Design review of the part built by this model. Coordinates are the model's own, in mm. A direction names the side the tool comes from. Coordinates: 2 decimals unless noted, no trailing zeros. Write each loop counter-clockwise with the first axis right and the second up, starting at its lowest first coordinate (ties: lowest second). Pieces come first, ordered by that corner, then holes.
Q1. For faces 1 (the flat face through (-17.58, 7.52, -11.09)), 2 (the flat face through (-28.001, 7.521, -11.476)), 3 (the flat face through (-12.3, 7.5, -3.8)), list the 3-axis set-ups (+Z, -Z, +X, -X, +Y, -Y) from which the entire face can be reached by the end or side of a thin tool; tool diameter is ignored.
Q2. Take a section at A-A, the plane x = -43. Write out the cut boundary in (y, z), plus the area to 3 significant figures.
Q3. For pin 1 Ø1.5 at (x, y) = (-40, 8) entering from -Z; pin 2 Ø1.5 at (x, y) = (-46.5, 7.5) entering from +Z; pin 3 Ø3 at (x, z) = (-23.15, -1.62) entering from -Y, all flat-tipped, find the tip position at first contact; note any pin that passes through.
Q4. Take a section at B-B, the plane y = 7.05. State how many separate pieces and enclosed holes the cut face has, plus the area to 3 significant figures.
Q5. For L1, parallel to X at y = 7.3, z = -9.25; L2, parallel to X at y = 6.2, z = -1.25; L3, parallel to Z at x = -38.5, y = 6.4, list the stretches that pass through material, from the lowest coordinate up.
Q6. The part is to be moulded in two halves that separate along Z. For faces 4 (the flat face through (-19.018, 7.521, -11.83)), 5 (the cylindrical face through (-21.785, 7.479, 8.289)), 6 (the flat face through (-29, 6, -2)), say which applies: released by +Z, released by -Z, zero draft, split by the parting line, or undercut.
from build123d import *

# Parameters (mm, degrees)
BOSS_EXTRUDE1_DEPTH   = 15
BOSS_EXTRUDE2_DEPTH   = 15
CIRPATTERN2_COUNT     = 13
CIRPATTERN2_ANGLE     = 170
F_1_0MM_DOWEL_HOLE1_D = 10
ESCALA1_SCALE         = 0.2


with BuildPart() as part:
    # Sketch1 → Boss-Extrude1 (new body)
    with BuildSketch(Plane(origin=(0, 0, 0), x_dir=(1, 0, 0), z_dir=(0, 1, 0))):
        with BuildLine():
            Line((-150, 15), (-47.696960071, 15))
            ThreePointArc((-47.696960071, 15), (50, 0), (-47.696960071, -15))
            Line((-47.696960071, -15), (-150, -15))
            ThreePointArc((-150, -15), (-165, 0), (-150, 15))
        make_face()
    extrude(amount=BOSS_EXTRUDE1_DEPTH)

    # Sketch2 → Boss-Extrude2 (add)
    with BuildSketch(Plane(origin=(0, 15, 0), x_dir=(1, 0, 0), z_dir=(0, 1, 0))):
        Polygon((49.877349569, 3.5), (60, 2), (60, -2), (49.877349569, -3.5), (50, 0), align=None)
    boss_extrude2 = extrude(amount=-BOSS_EXTRUDE2_DEPTH)

    # CirPattern2: Boss-Extrude2 ×13 about axis
    cirpattern2_axis = Axis((0, 0, 0), (0, 1, 0))
    for i in range(1, CIRPATTERN2_COUNT):
        add(boss_extrude2.rotate(cirpattern2_axis, i * CIRPATTERN2_ANGLE / (CIRPATTERN2_COUNT - 1)))

    # Ø1.0mm Dowel Hole1 (through all)
    with Locations(Plane(origin=(0, 15, 0), x_dir=(1, 0, 0), z_dir=(0, 1, 0))):
        with Locations((-150, 0), (0, 0)):
            Hole(F_1_0MM_DOWEL_HOLE1_D / 2)


with BuildPart() as part_1:
    # Escala1: scaled about (-28.934441086, 7.5, -2.022629068)
    add(part.part.scale(ESCALA1_SCALE).moved(Location((-23.147552869, 6, -1.618103254))))


solid = part_1.part
Responses:
1. face 1: -Z, +Y, -Y
1. face 2: +Y, -Y
1. face 3: +X, +Y, -Y
2. outline: (6, -4.62) - (9, -4.62) - (9, 1.38) - (6, 1.38) - close
2. area: 18.0 mm2
3. pin 1: stops at z = -4.62
3. pin 2: stops at z = 1.38
3. pin 3: stops at y = 6
4. separate pieces: 1
4. enclosed holes: 2
4. area: 469 mm2
5. L1: x = -32.41 to -32.1, -29.86 to -16.69, -15.71 to -14.18
5. L2: x = -56.12 to -54.08, -52.22 to -24.08, -22.22 to -11.15
5. L3: z = -4.62 to 1.38
6. face 4: undercut
6. face 5: released by +Z
6. face 6: zero draft
